Input: part model. Units: mm. Frame: model coordinates. A direction names the side the tool comes from. Coordinates: 2 decimals unless noted, no trailing zeros. Order: outer loops, then holes, each group sorted by start corner. A loop starts at its lowest first (then second) coordinate and runs counter-clockwise, first axis right, second up. Notation, with made-up numbers: (23, -19) - (33, -19) arc R23 ccw to (33, 13) - close; hole circle Ø10 at (-28, 86.25). An arc over 180 degrees is marked (long way). Answer as CSV lines item,"result". Start each with the question number.
Item 1: Section A-A (y = 49.5). Output: boundary loops of the cut face in (x, z), and give its area (3 significant figures).
Item 2: Draft query along Z for faces 1 (the flat face through (22.5, 42, 0)), 2 (the flat face through (0, 60, -20)), 3 (the flat face through (-5, 80, 0)). Return one class per face: +Z half, -Z half, draft (parallel to the pull), parting line (faces both ways), or undercut.
Item 3: First-contact query: pin 1 (10 mm diameter, centred on x = 13.5, y = 26, fed in from -Z); pin 2 (6 mm diameter, centred on x = 7, z = -3, fed in from +Y); pin 3 (5 mm diameter, centred on y = 16, z = 5, fed in from -X). Flat tips, straight axial feed; report the tip coordinate or a pass-through.
Item 4: Section D-D (y = 27). Output: boundary loops of the cut face in (x, z), and give its area (3 significant figures).
Item 5: Material intervals for line 1 along X through (y, z) = (2.75, 0); line 2 along Y through (x, z) = (-18, -16); line 3 along Z through (x, y) = (6, 66.5), sorted ascending.
Item 6: Access query for faces 4 (the cylindrical face through (-19.524, 19.72, -4.336)), 5 (the flat face through (0, 60, 20)), 6 (the flat face through (-1.5, 62, 0)), 7 (the flat face through (21, 40, 0)), 8 (the flat face through (-21, 40, 0)). Directions: +Z, -Z, +X, -X, +Y, -Y. A direction counts if a zero-diameter tool reaches every point of the face in a straight line with its end or side. Return the directions, or none.
Item 7: Section C-C (x = 12). Output: boundary loops of the cut face in (y, z).
Item 8: Section B-B (z = 0). Output: boundary loops of the cut face in (x, y), and give its area (3 significant figures).
from build123d import *

# Parameters (mm, degrees)
SKETCH1_R           = 20
BOSS_EXTRUDE1_DEPTH = 40
SKETCH2_R           = 2.7
CUT_EXTRUDE1_DEPTH  = 3.5
SKETCH3_W           = 40
SKETCH3_H           = 40
BOSS_EXTRUDE2_DEPTH = 25
SKETCH4_W           = 12.5
SKETCH4_H           = 40
CUT_EXTRUDE2_DEPTH  = 2.5
SKETCH5_W           = 12.5
SKETCH5_H           = 35.5
CUT_EXTRUDE3_DEPTH  = 24


with BuildPart() as part:
    # Sketch1 → Boss-Extrude1 (new body)
    with BuildSketch(Plane(origin=(0, 0, 0), x_dir=(1, 0, 0), z_dir=(0, 1, 0))):
        with Locations(Location((0, 0, 0), (0, 0, 270))):
            Circle(SKETCH1_R)
    extrude(amount=BOSS_EXTRUDE1_DEPTH)

    # Sketch2 → Cut-Extrude1 (cut)
    with BuildSketch(Plane.XZ):
        with Locations(Location((0, 0, 0), (0, 0, 270))):
            Circle(SKETCH2_R)
    extrude(amount=-CUT_EXTRUDE1_DEPTH, mode=Mode.SUBTRACT)

    # Sketch3 → Boss-Extrude2 (add, symmetric)
    with BuildSketch(Plane(origin=(0, 0, 0), x_dir=(0, 0, -1), z_dir=(1, 0, 0))):
        with Locations((0, 60)):
            Rectangle(SKETCH3_W, SKETCH3_H)
    extrude(amount=BOSS_EXTRUDE2_DEPTH, both=True)

    # Sketch4 → Cut-Extrude2 (cut)
    with BuildSketch(Plane(origin=(25, 0, 0), x_dir=(0, 0, -1), z_dir=(1, 0, 0))):
        with Locations((0, 60)):
            Rectangle(SKETCH4_W, SKETCH4_H)
    extrude(amount=-CUT_EXTRUDE2_DEPTH, mode=Mode.SUBTRACT)

    # Sketch5 → Cut-Extrude3 (cut)
    with BuildSketch(Plane(origin=(22.5, 0, 0), x_dir=(0, 0, -1), z_dir=(1, 0, 0))):
        with Locations((0, 62.25)):
            Rectangle(SKETCH5_W, SKETCH5_H)
    extrude(amount=-CUT_EXTRUDE3_DEPTH, mode=Mode.SUBTRACT)


solid = part.part
Determined:
1,outline,"(-25, -20) - (25, -20) - (25, -6.25) - (-1.5, -6.25) - (-1.5, 6.25) - (25, 6.25) - (25, 20) - (-25, 20) - close"
1,area,"1,670 mm^2"
2,face 1,"undercut"
2,face 2,"-Z half"
2,face 3,"draft"
3,pin 1,"stops at z = -18.1"
3,pin 2,"stops at y = 44.5"
3,pin 3,"stops at x = -19.84"
4,outline,"circle Ø40 at (0, 0)"
4,area,"1,260 mm^2"
5,line 1,"x = -20 to -2.7, 2.7 to 20"
5,line 2,"y = 40 to 80"
5,line 3,"z = -20 to -6.25, 6.25 to 20"
6,face 4,"-Y"
6,face 5,"+Z, +X, -X, +Y, -Y"
6,face 6,"+X, +Y"
6,face 7,"+X, -Y"
6,face 8,"-X, -Y"
7,outline,"(0, -16) - (40, -16) - (40, -20) - (80, -20) - (80, -6.25) - (44.5, -6.25) - (44.5, 6.25) - (80, 6.25) - (80, 20) - (40, 20) - (40, 16) - (0, 16) - close"
8,outline,"(-25, 40) - (-20, 40) - (-20, 0) - (-2.7, 0) - (-2.7, 3.5) - (2.7, 3.5) - (2.7, 0) - (20, 0) - (20, 40) - (22.5, 40) - (22.5, 44.5) - (-1.5, 44.5) - (-1.5, 80) - (-25, 80) - close"
8,area,"2,630 mm^2"
